Input: part model. Units: mm. Frame: model coordinates. A direction names the side the tool comes from. Round coordinates to 2 decimals unless told otherwise and drop trailing zeros. Order: outer loops, then holes, each group sorted by start corner. A loop starts at its lowest first (then second) coordinate and runs counter-clockwise, first axis right, second up. Notation, with made-up numbers: (9.25, 65.25) -> (45.25, 65.25) arc R36 cw to (45.25, 99.25) -> close; hole circle Ø7 at (62, 71.25). An arc over 180 degrees is marked (long way). Answer as CSV lines item,"result". Start each with the question number.
1) Section query B-B, the plane x = 54.5. Output: boundary loops of the cut face in (y, z).
2) Access query for faces 4 (the face through (92, 0, -71)), 5 (the face through (94, 186, -142)). Directions: +Z, -Z, +X, -X, +Y, -Y. A direction counts if a zero-diameter tool reaches every point of the face in a straight line with its end or side. Return the directions, or none.
3) Section query D-D, the plane y = 275. Output: boundary loops of the cut face in (x, z).
4) Line query: L1, parallel to Z at x = 80.5, y = 132; L2, parallel to X at y = 208, z = -141.4; L3, parallel to Y at x = 40, z = -141.65. Output: solid intervals per line, ascending.
5) Mould query, pull axis X, two halves, no side actions, for faces 1 (the face through (38.698, 89.915, 1.507)), 2 (the face through (2.96, 234.61, -141.51)), 3 (the face through (92, 145, 1)). Classes: +X half, -X half, draft (parallel to the pull), parting line (faces both ways), or undercut.
6) First-contact query: P1, Ø2, axis at x = 138, z = -26, coming from the +Y side. Flat tip, straight axial feed; report the tip coordinate or a pass-through.
7) Section query C-C, the plane z = -126.5. Output: boundary loops of the cut face in (x, y), and give its area (3 significant figures).
8) Section query A-A, the plane y = 138.5. Output: boundary loops of the cut face in (x, z), and give its area (3 significant figures).
```python
from build123d import *

# Parameters (mm, degrees)
SKETCH1_W                = 186.07
SKETCH1_H                = 140
BASE_FLANGE1_DEPTH       = 1
EDGE_FLANGE1_DEPTH       = 186.07
EDGE_FLANGE1_START       = 1
EDGE_FLANGE1_PROFILE_R   = 2.25
EDGE_FLANGE1_PROFILE_R_2 = 4.25
EDGE_FLANGE1_PROFILE_R_3 = 3.25
EDGE_FLANGE1_PROFILE_R_4 = 10
EDGE_FLANGE1_FLAT_DEPTH  = 1
EDGE_FLANGE2_DEPTH       = 186.07
EDGE_FLANGE2_START       = 1
EDGE_FLANGE2_PROFILE_R   = 3.25
EDGE_FLANGE2_PROFILE_R_2 = 10
EDGE_FLANGE2_PROFILE_R_3 = 2.25
EDGE_FLANGE2_PROFILE_R_4 = 4.25
EDGE_FLANGE2_FLAT_DEPTH  = 1
SKETCH21_R               = 1.5
CUT_EXTRUDE1_DEPTH       = 144


# Sheet-metal steps are written as plain solids
with BuildPart() as part:
    # Sketch1 → Base-Flange1 (new body)
    with BuildSketch(Plane(origin=(0, 0, 0), x_dir=(1, 0, 0), z_dir=(0, 1, 0))):
        with Locations((93.035, 70)):
            Rectangle(SKETCH1_W, SKETCH1_H)
    extrude(amount=-BASE_FLANGE1_DEPTH)

    # Edge-Flange1 bend section (across the edge) → Edge-Flange1 (add)
    with BuildSketch(Plane(origin=(0, 0, 1), x_dir=(0, 0, -1), z_dir=(1, 0, 0))):
        with BuildLine():
            Line((-1, 1), (0, 1))
            ThreePointArc((0, 1), (0.292893219, 0.292893219), (1, 0))
            Line((1, 0), (1, -1))
            ThreePointArc((1, -1), (-0.414213562, -0.414213562), (-1, 1))
        make_face()
    extrude(amount=EDGE_FLANGE1_DEPTH)

    # Edge-Flange1 profile (on flange) → Edge-Flange1 flat (add)
    with BuildSketch(Plane.XY.offset(1).offset(EDGE_FLANGE1_START)):
        with BuildLine():
            ThreePointArc((186.202497932, 325.709852824), (161.420468776, 362.701924453), (117.781829762, 353.857066198))
            Line((117.781829762, 353.857066198), (11.715746401, 247.791115203))
            ThreePointArc((11.715746401, 247.791115203), (3.044823475, 234.814175131), (0, 219.506826307))
            Line((0, 219.506826307), (0, 1))
            Line((0, 1), (186.202497932, 1))
            Line((186.202497932, 1), (186.202497932, 185.709852824))
            Line((186.202497932, 185.709852824), (186.202497932, 325.709852824))
        make_face()
        with Locations((146.20256152, 170.709852824)):
            Circle(EDGE_FLANGE1_PROFILE_R, mode=Mode.SUBTRACT)
        with Locations((161.20256152, 185.709852824)):
            Circle(EDGE_FLANGE1_PROFILE_R, mode=Mode.SUBTRACT)
        with Locations((146.202497932, 185.92936058)):
            Circle(EDGE_FLANGE1_PROFILE_R_2, mode=Mode.SUBTRACT)
        with Locations((131.20256152, 185.709852824)):
            Circle(EDGE_FLANGE1_PROFILE_R, mode=Mode.SUBTRACT)
        with Locations((67.5, 80)):
            Circle(EDGE_FLANGE1_PROFILE_R_3, mode=Mode.SUBTRACT)
        with Locations((40, 52.5)):
            Circle(EDGE_FLANGE1_PROFILE_R_3, mode=Mode.SUBTRACT)
        with Locations((40, 80)):
            Circle(EDGE_FLANGE1_PROFILE_R_4, mode=Mode.SUBTRACT)
        with Locations((12.5, 80)):
            Circle(EDGE_FLANGE1_PROFILE_R_3, mode=Mode.SUBTRACT)
        with Locations((40, 107.5)):
            Circle(EDGE_FLANGE1_PROFILE_R_3, mode=Mode.SUBTRACT)
        with Locations((146.20256152, 200.709852824)):
            Circle(EDGE_FLANGE1_PROFILE_R, mode=Mode.SUBTRACT)
        with Locations((146.2030357, 310.929360579)):
            Circle(EDGE_FLANGE1_PROFILE_R, mode=Mode.SUBTRACT)
        with Locations((161.203100232, 325.929360579)):
            Circle(EDGE_FLANGE1_PROFILE_R, mode=Mode.SUBTRACT)
        with Locations((146.203100232, 325.929360579)):
            Circle(EDGE_FLANGE1_PROFILE_R_2, mode=Mode.SUBTRACT)
        with Locations((146.203100232, 340.929360579)):
            Circle(EDGE_FLANGE1_PROFILE_R, mode=Mode.SUBTRACT)
        with Locations((131.203100232, 325.929360579)):
            Circle(EDGE_FLANGE1_PROFILE_R, mode=Mode.SUBTRACT)
    extrude(amount=-EDGE_FLANGE1_FLAT_DEPTH)

    # Edge-Flange2 bend section (across the edge) → Edge-Flange2 (add)
    with BuildSketch(Plane(origin=(186.07, 0, -141), x_dir=(0, 0, 1), z_dir=(-1, 0, 0))):
        with BuildLine():
            Line((-1, 1), (0, 1))
            ThreePointArc((0, 1), (0.292893219, 0.292893219), (1, 0))
            Line((1, 0), (1, -1))
            ThreePointArc((1, -1), (-0.414213562, -0.414213562), (-1, 1))
        make_face()
    extrude(amount=EDGE_FLANGE2_DEPTH)

    # Edge-Flange2 profile (on flange) → Edge-Flange2 flat (add)
    with BuildSketch(Plane(origin=(0, 0, -141), x_dir=(-1, 0, 0), z_dir=(0, 0, -1)).offset(EDGE_FLANGE2_START)):
        with BuildLine():
            ThreePointArc((-117.781829762, 353.857066198), (-161.347263599, 362.640665891), (-186.07, 325.709852824))
            Line((-186.07, 325.709852824), (-186.07, 1))
            Line((-186.07, 1), (0, 1))
            Line((0, 1), (0, 219.506826307))
            ThreePointArc((0, 219.506826307), (-3.044823475, 234.814175131), (-11.715746401, 247.791115203))
            Line((-11.715746401, 247.791115203), (-117.781829762, 353.857066198))
        make_face()
        with Locations((-12.5, 80)):
            Circle(EDGE_FLANGE2_PROFILE_R, mode=Mode.SUBTRACT)
        with Locations((-40, 52.5)):
            Circle(EDGE_FLANGE2_PROFILE_R, mode=Mode.SUBTRACT)
        with Locations((-40, 80)):
            Circle(EDGE_FLANGE2_PROFILE_R_2, mode=Mode.SUBTRACT)
        with Locations((-40, 107.5)):
            Circle(EDGE_FLANGE2_PROFILE_R, mode=Mode.SUBTRACT)
        with Locations((-67.5, 80)):
            Circle(EDGE_FLANGE2_PROFILE_R, mode=Mode.SUBTRACT)
        with Locations((-131.20256152, 185.709852824)):
            Circle(EDGE_FLANGE2_PROFILE_R_3, mode=Mode.SUBTRACT)
        with Locations((-146.20256152, 170.709852824)):
            Circle(EDGE_FLANGE2_PROFILE_R_3, mode=Mode.SUBTRACT)
        with Locations((-146.202497932, 185.92936058)):
            Circle(EDGE_FLANGE2_PROFILE_R_4, mode=Mode.SUBTRACT)
        with Locations((-161.20256152, 185.709852824)):
            Circle(EDGE_FLANGE2_PROFILE_R_3, mode=Mode.SUBTRACT)
        with Locations((-146.20256152, 200.709852824)):
            Circle(EDGE_FLANGE2_PROFILE_R_3, mode=Mode.SUBTRACT)
        with Locations((-131.203100232, 325.929360579)):
            Circle(EDGE_FLANGE2_PROFILE_R_3, mode=Mode.SUBTRACT)
        with Locations((-146.2030357, 310.929360579)):
            Circle(EDGE_FLANGE2_PROFILE_R_3, mode=Mode.SUBTRACT)
        with Locations((-146.125015413, 325.709852824)):
            Circle(EDGE_FLANGE2_PROFILE_R_4, mode=Mode.SUBTRACT)
        with Locations((-146.203100232, 340.929360579)):
            Circle(EDGE_FLANGE2_PROFILE_R_3, mode=Mode.SUBTRACT)
        with Locations((-161.203100232, 325.929360579)):
            Circle(EDGE_FLANGE2_PROFILE_R_3, mode=Mode.SUBTRACT)
    extrude(amount=-EDGE_FLANGE2_FLAT_DEPTH)

    # Sketch21 → Cut-Extrude1 (cut)
    with BuildSketch(Plane(origin=(0, 0, -142), x_dir=(-1, 0, 0), z_dir=(0, 0, -1))):
        with Locations(Location((-181.07, 118, 0), (0, 0, 90))):
            Circle(SKETCH21_R)
        with Locations(Location((-181.07, 168, 0), (0, 0, 90))):
            Circle(SKETCH21_R)
        with Locations(Location((-181.07, 68, 0), (0, 0, 90))):
            Circle(SKETCH21_R)
        with Locations(Location((-181.07, 208, 0), (0, 0, 90))):
            Circle(SKETCH21_R)
        with Locations(Location((-181.07, 258, 0), (0, 0, 90))):
            Circle(SKETCH21_R)
        with Locations(Location((-181.07, 308, 0), (0, 0, 90))):
            Circle(SKETCH21_R)
    extrude(amount=-CUT_EXTRUDE1_DEPTH, mode=Mode.SUBTRACT)


solid = part.part
```
Findings:
1,outline,"(-1, -140) arc R2 ccw to (1, -142) -> (290.58, -142) -> (290.58, -141) -> (1, -141) arc R1 cw to (0, -140) -> (0, 0) arc R1 cw to (1, 1) -> (290.58, 1) -> (290.58, 2) -> (1, 2) arc R2 ccw to (-1, 0) -> close"
2,face 4,"+X, -X, +Y"
2,face 5,"-Z, +X, -X, +Y, -Y"
3,outline,"(38.92, -142) -> (186.07, -142) -> (186.07, -141) -> (38.92, -141) -> close; (38.92, 1) -> (186.2, 1) -> (186.2, 2) -> (38.92, 2) -> close"
4,L1,"z = -142 to -141, 1 to 2"
4,L2,"x = 0 to 179.57, 182.57 to 186.07"
4,L3,"y = -0.13 to 49.25, 55.75 to 70, 90 to 104.25, 110.75 to 276.08"
5,face 1,"undercut"
5,face 2,"-X half"
5,face 3,"draft"
6,P1,"stops at y = 0"
7,outline,"(0, -1) -> (186.07, -1) -> (186.07, 0) -> (0, 0) -> close"
7,area,"186 mm^2"
8,outline,"(0, -142) -> (186.07, -142) -> (186.07, -141) -> (0, -141) -> close; (0, 1) -> (186.2, 1) -> (186.2, 2) -> (0, 2) -> close"
8,area,"372 mm^2"
